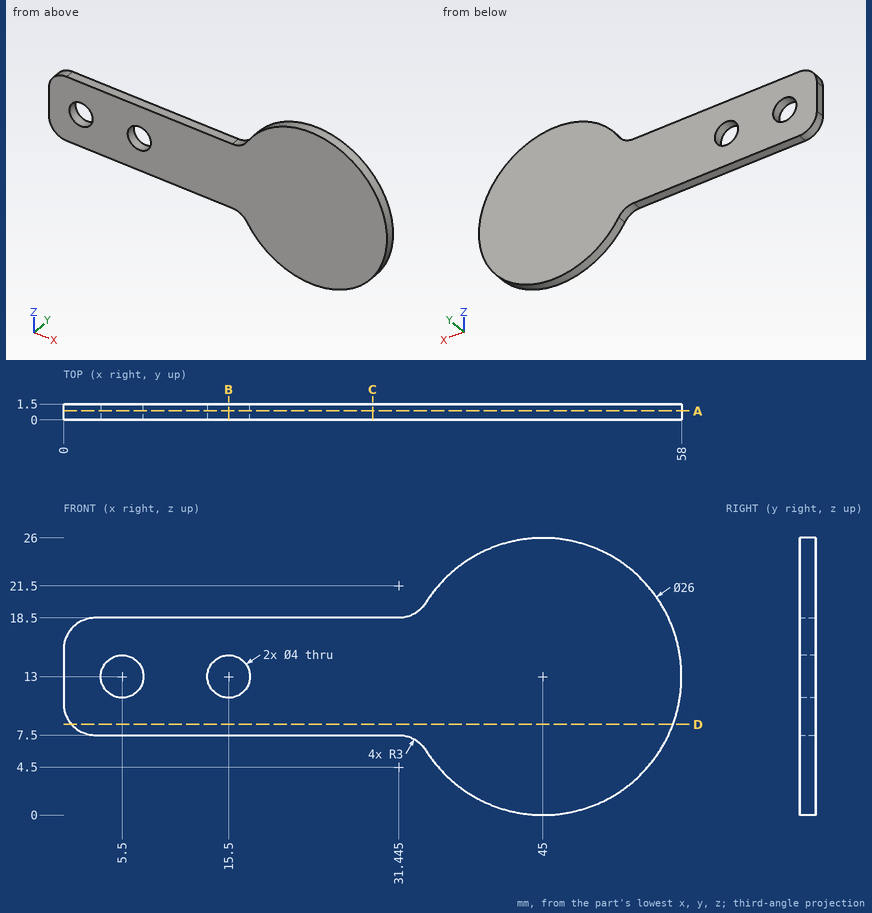
Job drawing, mm, ordinate dimensions from the low corner. One solid piece. Give positions to 0.01 mm unless a question says otherwise; leave off trailing zeros. Loops run counter-clockwise (first coordinate to the right, second up) from the corner with the lowest first, then second, coordinate; pieces in that order, holes last. Notation, with made-up numbers: M -13,46 L 43,46 A16 cw 43,66 Z; hole C 34.25,5 d6. An arc over 180 degrees is marked long. Answer in a Markdown table with one row per item. Add a question column.
Item 1: Drop flat-ended pins along their axis: P1, Ø12, axis at x = 19.5, z = 5, coming from the +Y side; P2, Ø0.8, axis at x = 14, y = 0.5, coming from the -Z side. Give the stop position or say it passes through.
Item 2: Band-saw the part on B-B on x = 15.5. Give the cut face in (y, z), then the cut area to 3 significant figures.
Item 3: Band-saw the part on D-D on z = 8.5. Give the cut face in (x, y).
Item 4: Probe probe 1 along Z at (x, y) = (15.5, 0.45); probe 2 along X at (y, z) = (0.4, 14.5) (1 decimal); probe 3 along X at (y, z) = (0.5, 11.75). List the from-to ranges inside material, lowest first.
Item 5: Band-saw the part on C-C on x = 29. Give the cut face in (y, z), then the cut area to 3 significant figures.
Item 6: Band-saw the part on A-A on y = 0.85. Give the cut face in (x, z) (1 decimal).
Reply:
| question | item | result |
|---|---|---|
| 1 | P1 | stops at y = 1.5 |
| 1 | P2 | stops at z = 7.5 |
| 2 | outline | M 0,7.5 L 1.5,7.5 L 1.5,11 L 0,11 Z; M 0,15 L 1.5,15 L 1.5,18.5 L 0,18.5 Z |
| 2 | area | 10.5 mm^2 |
| 3 | outline | M 0.76,0 L 57.2,0 L 57.2,1.5 L 0.76,1.5 Z |
| 4 | probe 1 | z = 7.5 to 11, 15 to 18.5 |
| 4 | probe 2 | x = 0 to 4.2, 6.8 to 14.2, 16.8 to 57.9 |
| 4 | probe 3 | x = 0 to 3.94, 7.06 to 13.94, 17.06 to 57.94 |
| 5 | outline | M 0,7.5 L 1.5,7.5 L 1.5,18.5 L 0,18.5 Z |
| 5 | area | 16.5 mm^2 |
| 6 | outline | M 0,10.5 A3 ccw 3,7.5 L 31.4,7.5 A3 cw 34,6.1 A13 ccw long 34,19.9 A3 cw 31.4,18.5 L 3,18.5 A3 ccw 0,15.5 Z; hole C 5.5,13 d4; hole C 15.5,13 d4 |
